Part model, mm, in its own coordinate system. A direction names the side the tool comes from. Round coordinates to 2 decimals unless told otherwise and drop trailing zeros. Order: outer loops, then holes, each group sorted by start corner. A loop starts at its lowest first (then second) coordinate and runs counter-clockwise, first axis right, second up. Notation, with made-up numbers: (-10, 4.25) -> (9, 4.25) arc R22 cw to (9, 36.25) -> close; hole circle Ø8 at (-15, 75.25). An arc over 180 degrees is marked (long way). Answer as a JSON object with one key per item and string values. Group by question number.
```python
from build123d import *

# Parameters (mm, degrees)
SKETCH1_W           = 88.9
SKETCH1_H           = 30.48
BOSS_EXTRUDE1_DEPTH = 3.175
SKETCH3_W           = 5.08
SKETCH3_H           = 3.175
BOSS_EXTRUDE2_DEPTH = 3.175
SKETCH4_W           = 5.08
SKETCH4_H           = 3.175
BOSS_EXTRUDE3_DEPTH = 3.175
SKETCH5_W           = 6.35
SKETCH5_H           = 5.08
BOSS_EXTRUDE4_DEPTH = 3.175


with BuildPart() as part:
    # Sketch1 → Boss-Extrude1 (new body)
    with BuildSketch(Plane(origin=(0, 0, 0), x_dir=(1, 0, 0), z_dir=(0, 1, 0))):
        Rectangle(SKETCH1_W, SKETCH1_H)
    extrude(amount=BOSS_EXTRUDE1_DEPTH)

    # Sketch3 → Boss-Extrude2 (add)
    with BuildSketch(Plane(origin=(0, 0, 0), x_dir=(1, 0, 0), z_dir=(0, 1, 0))):
        with Locations((-25.4, -16.8275)):
            Rectangle(SKETCH3_W, SKETCH3_H)
        with Locations((-15.24, -16.8275)):
            Rectangle(SKETCH3_W, SKETCH3_H)
        with Locations((-5.08, -16.8275)):
            Rectangle(SKETCH3_W, SKETCH3_H)
        with Locations((5.08, -16.8275)):
            Rectangle(SKETCH3_W, SKETCH3_H)
        with Locations((15.24, -16.8275)):
            Rectangle(SKETCH3_W, SKETCH3_H)
        with Locations((25.4, -16.8275)):
            Rectangle(SKETCH3_W, SKETCH3_H)
    extrude(amount=BOSS_EXTRUDE2_DEPTH)

    # Sketch4 → Boss-Extrude3 (add)
    with BuildSketch(Plane(origin=(0, 3.175, 0), x_dir=(1, 0, 0), z_dir=(0, 1, 0))):
        with Locations((-25.4, -20.0025)):
            Rectangle(SKETCH4_W, SKETCH4_H)
        with Locations((-15.24, -20.0025)):
            Rectangle(SKETCH4_W, SKETCH4_H)
        with Locations((-5.08, -20.0025)):
            Rectangle(SKETCH4_W, SKETCH4_H)
        with Locations((5.08, -20.0025)):
            Rectangle(SKETCH4_W, SKETCH4_H)
        with Locations((15.24, -20.0025)):
            Rectangle(SKETCH4_W, SKETCH4_H)
        with Locations((25.4, -20.0025)):
            Rectangle(SKETCH4_W, SKETCH4_H)
    extrude(amount=-BOSS_EXTRUDE3_DEPTH)

    # Sketch5 → Boss-Extrude4 (add)
    with BuildSketch(Plane(origin=(0, 3.175, 0), x_dir=(1, 0, 0), z_dir=(0, 1, 0))):
        with Locations((-47.625, 2.54)):
            Rectangle(SKETCH5_W, SKETCH5_H)
        with Locations((-47.625, 12.7)):
            Rectangle(SKETCH5_W, SKETCH5_H)
        with Locations((-47.625, -7.62)):
            Rectangle(SKETCH5_W, SKETCH5_H)
        with Locations((47.625, -7.62)):
            Rectangle(SKETCH5_W, SKETCH5_H)
        with Locations((47.625, 2.54)):
            Rectangle(SKETCH5_W, SKETCH5_H)
        with Locations((47.625, 12.7)):
            Rectangle(SKETCH5_W, SKETCH5_H)
    extrude(amount=-BOSS_EXTRUDE4_DEPTH)


solid = part.part
```
Q1. Wall check: line 1 (X direction, y = 2.2, z = 16.5); line 2 (Z direction, x = 46.5, y = 0.3); line 3 (Z direction, x = 1.5, y = 1.5). Give the ranges that are in metal, low to high. Write a range as [from, to].
Q2. Two-plate mould, pull along Z, no slides. Class faces 1 (the flat face through (25, 2, 21.59)), 2 (the flat face through (12.7, 2, 18)), 3 (the flat face through (-48, 2, -5.08)): +Z half, -Z half, draft (parallel to the pull), parting line (faces both ways), or undercut.
Q3. Band-saw the part on A-A (z = 1). List the corners of the cut face in (x, y) (3 decimals), plus the area to 3 significant figures.
Q4. Drop flat-ended pins along their axis: pin 1 Ø1 at (x, y) = (37.5, 1.5) entering from +Z; pin 2 Ø1 at (y, z) = (1, 2) entering from +X; pin 3 Ø1.6 at (x, y) = (-47, 2) entering from +Z. Give the stop position or say it passes through.
Q5. Band-saw the part on B-B (x = 37.5). List the corners of the cut face in (y, z) (3 decimals), plus the area to 3 significant figures.
Q6. Which spindle directions (+Z, -Z, +X, -X, +Y, -Y) get a long thin tool onto all of the face, cutting with end or side? Do faces 4 (the flat face through (36, 2, 15.24)), 5 (the flat face through (-7.62, 2, 18)), 6 (the flat face through (48, 2, -5.08)). Say none if no direction does.
Completed:
{
 "1": {"line 1": "[-27.94, -22.86], [-17.78, -12.7], [-7.62, -2.54], [2.54, 7.62], [12.7, 17.78], [22.86, 27.94]", "line 2": "[-15.24, -10.16], [-5.08, 0], [5.08, 10.16]", "line 3": "[-15.24, 15.24]"},
 "2": {"face 1": "+Z half", "face 2": "draft", "face 3": "undercut"},
 "3": {"outline": "(-44.45, 0) -> (44.45, 0) -> (44.45, 3.175) -> (-44.45, 3.175) -> close", "area": "282 mm2"},
 "4": {"pin 1": "z = 15.24", "pin 2": "x = 44.45", "pin 3": "z = 10.16"},
 "5": {"outline": "(0, -15.24) -> (3.175, -15.24) -> (3.175, 15.24) -> (0, 15.24) -> close", "area": "96.8 mm2"},
 "6": {"face 4": "+Z, +X, +Y, -Y", "face 5": "+Z, +Y, -Y", "face 6": "+X, +Y, -Y"}
}
